```python
from build123d import *

# Parameters (mm, degrees)
CYLINDER1388_R     = 1.7
CYLINDER1388_DEPTH = 1
CYLINDER1386_R     = 3.5
CYLINDER1386_DEPTH = 1


with BuildPart() as cylinder1388:
    # Cylinder1388 → Cylinder1388 (new body)
    with BuildSketch(Plane(origin=(436, 103, 100), x_dir=(0, 0, -1), z_dir=(1, 0, 0))):
        Circle(CYLINDER1388_R)
    extrude(amount=CYLINDER1388_DEPTH)


with BuildPart() as bucket_left_half_short_spacer:
    # Cylinder1386 → Cylinder1386 (new body)
    with BuildSketch(Plane(origin=(436, 103, 100), x_dir=(0, 0, -1), z_dir=(1, 0, 0))):
        Circle(CYLINDER1386_R)
    extrude(amount=CYLINDER1386_DEPTH)

    # Cut014355: cut Cylinder1388
    add(cylinder1388.part, mode=Mode.SUBTRACT)


with BuildPart() as bucket_left_half_short_spacer_1:
    # Cut014355 placement: moved
    add(bucket_left_half_short_spacer.part.moved(Location((-0.5, 0, 0))))


solid = bucket_left_half_short_spacer_1.part
```
Verification items for the finished model (mm, model axes). Round coordinates to 2 decimals unless told otherwise and drop trailing zeros. Order: outer loops, then holes, each group sorted by start corner. A loop starts at its lowest first (then second) coordinate and runs counter-clockwise, first axis right, second up. Notation, with made-up numbers: (-40, 11) - (-16, 11) arc R24 ccw to (-16, 24) - close; hole circle Ø3 at (69.25, 76.25). An arc over 180 degrees is marked (long way). Use CSV: the item, a comma, the result in double quotes.
(1) Section check C-C on x = 436.4. Record the boundary of the cut face in (y, z), and give its area (3 significant figures).
Entries:
outline,"circle Ø7 at (103, 100); hole circle Ø3.4 at (103, 100)"
area,"29.4 mm^2"
(2) Thickness scan on probe 1 along Y at (x, z) = (435.85, 100); probe 2 along Z at (x, y) = (436.35, 104.25); probe 3 along Y at (x, z) = (436.15, 101.25). Record the ranges inside material, lowest first. Write a range as from..to.
Entries:
probe 1,"99.5..101.3, 104.7..106.5"
probe 2,"96.73..98.85, 101.15..103.27"
probe 3,"99.73..101.85, 104.15..106.27"
(3) Section check D-D on z = 97.75. Record the boundary of the cut face in (x, y), and give its area (3 significant figures).
Entries:
outline,"(435.5, 100.32) - (436.5, 100.32) - (436.5, 105.68) - (435.5, 105.68) - close"
area,"5.36 mm^2"
(4) Section check A-A on y = 103. Record the boundary of the cut face in (x, z).
Entries:
outline,"(435.5, 96.5) - (436.5, 96.5) - (436.5, 98.3) - (435.5, 98.3) - close; (435.5, 101.7) - (436.5, 101.7) - (436.5, 103.5) - (435.5, 103.5) - close"
(5) Mould release check, pull along Y, two halves, no side actions. Record for faces 1 (the face through (435.99, 101.97, 101.35)), 2 (the face through (435.993, 101.659, 96.767)), 3 (the face through (435.5, 104, 98)): released by +Y, released by -Y, zero draft, split by the parting line, or undercut.
Entries:
face 1,"undercut"
face 2,"split by the parting line"
face 3,"zero draft"
(6) Section check B-B on z = 100. Record the boundary of the cut face in (x, y).
Entries:
outline,"(435.5, 99.5) - (436.5, 99.5) - (436.5, 101.3) - (435.5, 101.3) - close; (435.5, 104.7) - (436.5, 104.7) - (436.5, 106.5) - (435.5, 106.5) - close"
